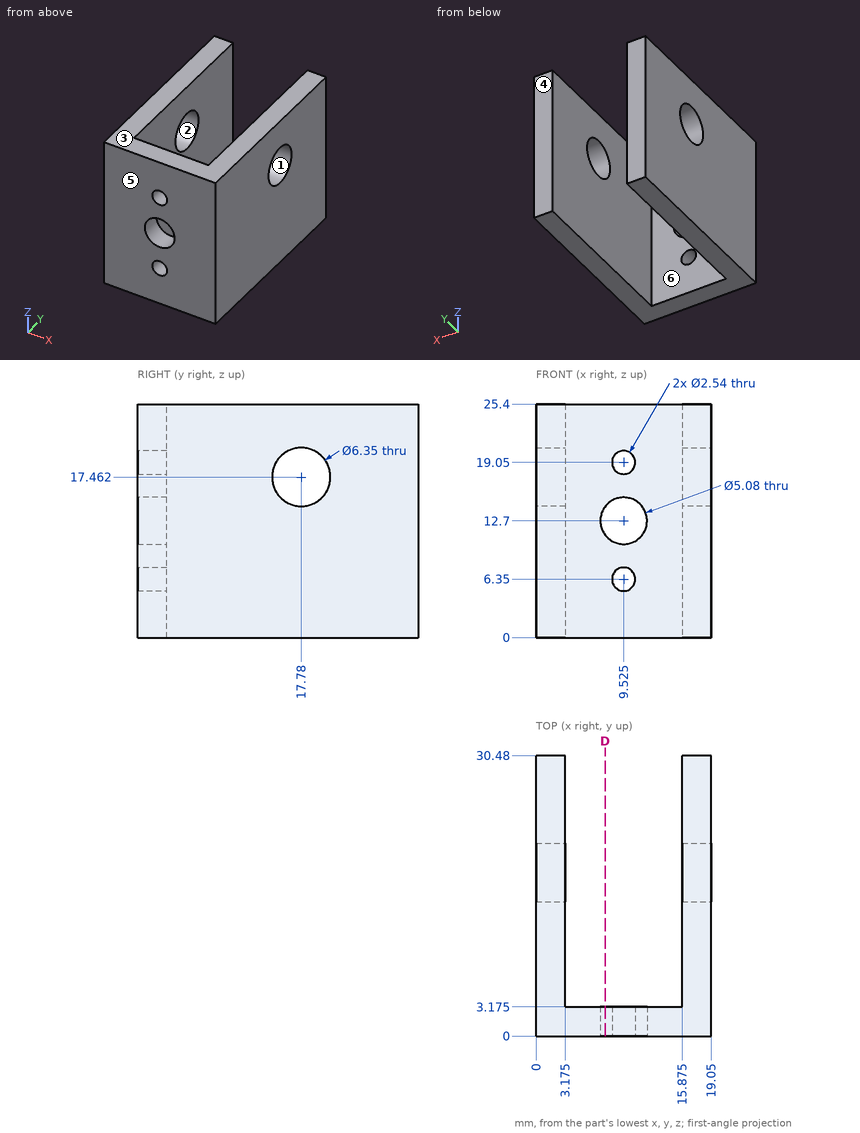
Geometry check sheet. Reference: drawing and pictorial views, mm from the part's lowest x, y, z. A direction names the side the tool comes from. Round coordinates to 2 decimals unless told otherwise and drop trailing zeros. Write each loop counter-clockwise with the first axis right and the second up, starting at its lowest first coordinate (ties: lowest second). Pieces come first, ordered by that corner, then holes.
1. Scan lines: L1, parallel to Y at x = 14.5, z = 16 (1 decimal); L2, parallel to Y at x = 2.5, z = 19. Record each from-to range of solid material in increasing order.
2. Draft check along Z on the marked faces 1, 2, 3 and 4. Enter one of: +Z half, -Z half, draft (parallel to the pull), parting line (faces both ways), or undercut.
3. Gauge pin test, flat ends, axial feed: P1, Ø5, axis at x = 9.5, z = 12, coming from the +Y side (1 decimal); P2, Ø2, axis at x = 5, y = 12.5, coming from the +Z side. Record the tip position at first contact, or that the pin passes through.
4. Section check D-D on x = 7.5. Enter the section's corners in (y, z) (1 decimal).
5. Access from +Z, -Z, +X, -X, +Y, -Y to the whole of each face (thin tool, end or side, straight path). Record for the marked faces 5 and 6.
Answer:
1. L1: y = 0 to 3.2
1. L2: y = 0 to 15, 20.56 to 30.48
2. face 1: undercut
2. face 2: undercut
2. face 3: +Z half
2. face 4: draft
3. P1: stops at y = 3.2
3. P2: passes through
4. outline: (0, 0) - (3.2, 0) - (3.2, 11.2) - (0, 11.2) - close; (0, 14.2) - (3.2, 14.2) - (3.2, 25.4) - (0, 25.4) - close
5. face 5: +Z, -Z, +X, -X, -Y
5. face 6: +Z, -Z, +Y
